Verification items for this drawing (mm, ordinates from the low corner). Round coordinates to 2 decimals unless told otherwise and drop trailing zeros. Loops run counter-clockwise (first coordinate to the right, second up) from the corner with the lowest first, then second, coordinate; pieces in that order, holes last. Notation, with made-up numbers: (38.25, 75) - (88.25, 75) arc R22 cw to (88.25, 103) - close; hole circle Ø3 at (84, 22.5). An arc over 180 degrees is marked (long way). Put each result on its own line as item: value.
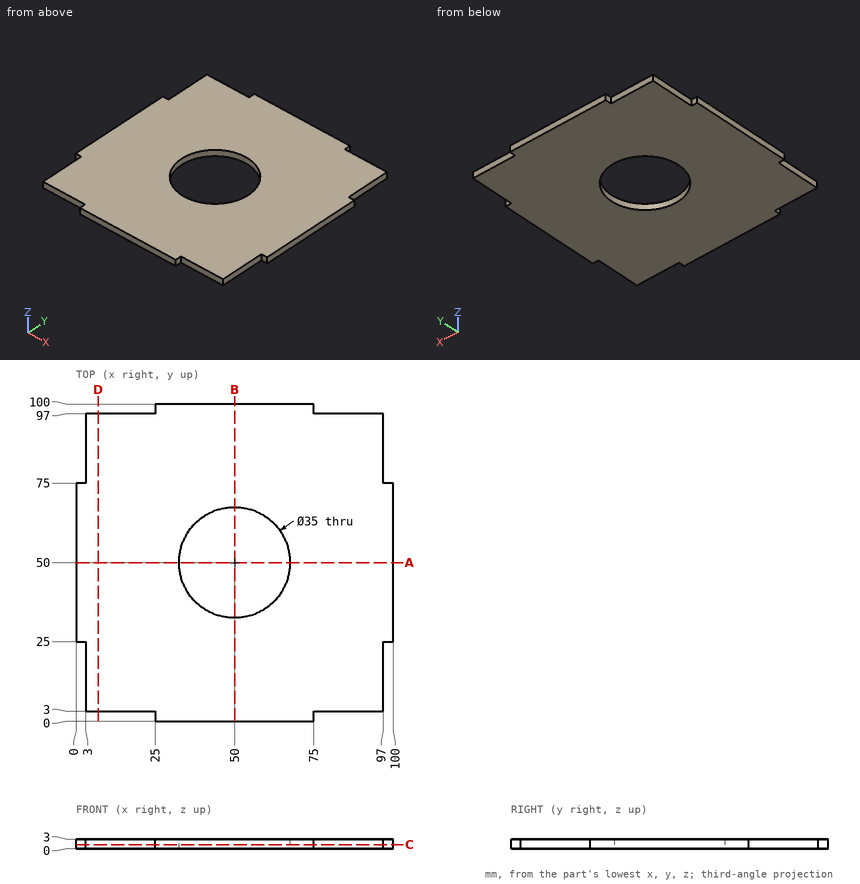
Item 1: Go/stop test with flat-tipped pins: pin 1 (1.5 mm diameter, centred on x = 80.5, z = 2, fed in from -Y); pin 2 (3 mm diameter, centred on x = 15.5, y = 60.5, fed in from -Z); pin 3 (1.5 mm diameter, centred on x = 88.5, z = 2, fed in from +Y); pin 4 (21 mm diameter, centred on x = 50, y = 50, fed in from -Z). Record where each tip stops, or that it passes through.
Filled sheet:
pin 1: y = 3
pin 2: z = 0
pin 3: y = 97
pin 4: through
Item 2: Thickness scan on line 1 (Y direction, x = 50, z = 2.15); line 2 (Y direction, x = 95.5, z = 2.3). Record the ranges inside material, lowest first. Write a range as from..to.
Filled sheet:
line 1: 0..32.5, 67.5..100
line 2: 3..97
Item 3: Section check D-D on x = 7. Enter the section's corners in (y, z).
Filled sheet:
outline: (3, 0) - (97, 0) - (97, 3) - (3, 3) - close
Item 4: Section check A-A on y = 50. Enter the section's corners in (x, z), then the cut area to 3 significant figures.
Filled sheet:
outline: (0, 0) - (32.5, 0) - (32.5, 3) - (0, 3) - close; (67.5, 0) - (100, 0) - (100, 3) - (67.5, 3) - close
area: 195 mm²
Item 5: Section check C-C on z = 1.2. Enter the section's corners in (x, y).
Filled sheet:
outline: (0, 25) - (3, 25) - (3, 3) - (25, 3) - (25, 0) - (75, 0) - (75, 3) - (97, 3) - (97, 25) - (100, 25) - (100, 75) - (97, 75) - (97, 97) - (75, 97) - (75, 100) - (25, 100) - (25, 97) - (3, 97) - (3, 75) - (0, 75) - close; hole circle Ø35 at (50, 50)
